Could you check a few things on this model? Use its own coordinates, in mm. A direction names the side the tool comes from. Give positions to 0.01 mm unless a question says otherwise; leave off trailing zeros. Order: outer loops, then holes, each group sorted by start corner. A loop starts at its lowest first (then second) coordinate and runs counter-clockwise, first axis right, second up. Notation, with made-up numbers: M 72,15.5 L 125,15.5 A20 ccw 125,21.5 Z; hole C -1.75,71 d11. An arc over 180 degrees is marked long. Answer in a Markdown table with one row per item. Add a question column.
```python
from build123d import *

# Parameters (mm, degrees)
SKETCH3_W           = 7.302665
SKETCH3_H           = 36.305572
FACE_CUT_DEPTH      = 10
LINK_ARMS_REACH     = 26.639
ROUNDED_LINKS_REACH = 32.365
SKETCH6_R           = 4
TRIM_1_REACH        = 35.167
SKETCH7_R           = 1.5
SKETCH8_W           = 8
SKETCH8_H           = 8.25
TRIM_2_DEPTH        = 15


with BuildPart() as part:
    # Sketch1 → Base Cylinder (revolve)
    with BuildSketch(Plane.XY, mode=Mode.PRIVATE) as base_cylinder_sk:
        with BuildLine():
            Line((-16, 2.5), (-16, 7.5))
            Line((-16, 7.5), (-12.5, 7.5))
            ThreePointArc((-12.5, 7.5), (-11.792893, 7.792893), (-11.5, 8.5))
            Line((-11.5, 8.5), (-11.5, 9.75))
            Line((-11.5, 9.75), (0, 9.75))
            Line((0, 9.75), (0, 8.25))
            Line((0, 8.25), (-3.5, 8.25))
            Line((-3.5, 8.25), (-3.5, 2.5))
            Line((-3.5, 2.5), (-16, 2.5))
        make_face()
    revolve(base_cylinder_sk.sketch.rotate(Axis((-29.02439, 0, 0), (1, 0, 0)), 90), axis=Axis((-29.02439, 0, 0), (1, 0, 0)))

    # Sketch2 → Suspension attachments (revolve)
    with BuildSketch(Plane(origin=(-3.375, 0, 0), x_dir=(0, 0, -1), z_dir=(1, 0, 0))):
        with BuildLine():
            Line((-3.375, 16), (-1.5, 16))
            Line((-1.5, 16), (-1.5, 9.633924))
            ThreePointArc((-1.5, 9.633924), (-3.80208, 8.978123), (-5.875, 7.781187))
            Line((-5.875, 7.781187), (-3.375, 12.111314))
            Line((-3.375, 12.111314), (-3.375, 16))
        make_face()
    suspension_attachments = revolve(axis=Axis((-3.375, 16.888615, 0), (0, -1, 0)))

    # Mirror1: Suspension attachments across plane
    add(suspension_attachments.mirror(Plane.ZX))

    # Sketch3 → Face Cut (cut, symmetric)
    with BuildSketch(Plane.XY):
        with Locations((3.651332, -0.216492)):
            Rectangle(SKETCH3_W, SKETCH3_H)
    extrude(amount=FACE_CUT_DEPTH, both=True, mode=Mode.SUBTRACT)

    # Link Arms: up to this face of the body (flat: up to its plane)
    link_arms_end = Plane(part.part.faces().sort_by_distance((-11.5, 0, -8.775772))[0])
    # Sketch5 → Link Arms (add, up to the picked face)
    with BuildSketch(Plane(origin=(0, 0, 0), x_dir=(0, 0, -1), z_dir=(1, 0, 0)), mode=Mode.PRIVATE) as link_arms_sk1:
        with BuildLine():
            Line((9.75, 0), (20.25, 0))
            Line((20.25, 0), (20.25, -2.5))
            Line((20.25, -2.5), (9.424038, -2.5))
            ThreePointArc((9.424038, -2.5), (9.668166, -1.26058), (9.75, 0))
        make_face()
    link_arms_tool1 = split(extrude(link_arms_sk1.sketch, amount=-LINK_ARMS_REACH, mode=Mode.PRIVATE), bisect_by=link_arms_end, keep=Keep.BOTH, mode=Mode.PRIVATE)
    # Sketch5 → Link Arms (add, up to the picked face)
    with BuildSketch(Plane(origin=(0, 0, 0), x_dir=(0, 0, -1), z_dir=(1, 0, 0)), mode=Mode.PRIVATE) as link_arms_sk2:
        with BuildLine():
            Line((5.887009, -7.772106), (11.044873, -10.75))
            Line((11.044873, -10.75), (20.25, -10.75))
            Line((20.25, -10.75), (20.25, -13.25))
            Line((20.25, -13.25), (10.375, -13.25))
            Line((10.375, -13.25), (3.309929, -9.17098))
            ThreePointArc((3.309929, -9.17098), (4.651358, -8.568977), (5.887009, -7.772106))
        make_face()
    link_arms_tool2 = split(extrude(link_arms_sk2.sketch, amount=-LINK_ARMS_REACH, mode=Mode.PRIVATE), bisect_by=link_arms_end, keep=Keep.BOTH, mode=Mode.PRIVATE)
    add(link_arms_tool1.solids().sort_by(Axis((0, -1.25638, -14.945599), (-1, 0, 0)))[0])
    add(link_arms_tool2.solids().sort_by(Axis((0, -11.294384, -12.172928), (-1, 0, 0)))[0])

    # Rounded Links: up to this face of the body (flat: up to its plane)
    rounded_links_end = Plane(part.part.faces().sort_by_distance((-5.75, -13.25, -15.3125))[0])
    # Sketch6 → Rounded Links (add, up to the picked face)
    with BuildSketch(Plane(origin=(0, 0, 0), x_dir=(1, 0, 0), z_dir=(0, 1, 0)), mode=Mode.PRIVATE) as rounded_links_sk1:
        with Locations(Location((-5.75, 20.25, 0), (0, 0, 180))):
            Circle(SKETCH6_R)
    rounded_links_tool1 = split(extrude(rounded_links_sk1.sketch, amount=-ROUNDED_LINKS_REACH, mode=Mode.PRIVATE), bisect_by=rounded_links_end, keep=Keep.BOTH, mode=Mode.PRIVATE)
    add(rounded_links_tool1.solids().sort_by(Axis((-5.75, 0, -20.25), (0, -1, 0)))[0])

    # Trim 1: up to this face of the body (flat: up to its plane)
    trim_1_end = Plane(part.part.faces().sort_by_distance((-5.75, -13.25, -16.514845))[0])
    # Sketch7 → Trim 1 (cut, up to the picked face)
    with BuildSketch(Plane(origin=(0, 0, 0), x_dir=(1, 0, 0), z_dir=(0, 1, 0)), mode=Mode.PRIVATE) as trim_1_sk1:
        with Locations(Location((-5.75, 20.25, 0), (0, 0, 270))):
            Circle(SKETCH7_R)
    trim_1_tool1 = split(extrude(trim_1_sk1.sketch, amount=-TRIM_1_REACH, mode=Mode.PRIVATE), bisect_by=trim_1_end, keep=Keep.BOTH, mode=Mode.PRIVATE)
    # Sketch7 → Trim 1 (cut, up to the picked face)
    with BuildSketch(Plane(origin=(0, 0, 0), x_dir=(1, 0, 0), z_dir=(0, 1, 0)), mode=Mode.PRIVATE) as trim_1_sk2:
        Polygon((-9.75, 20.25), (-11.5, 9.75), (-11.5, 20.25), align=None)
    trim_1_tool2 = split(extrude(trim_1_sk2.sketch, amount=-TRIM_1_REACH, mode=Mode.PRIVATE), bisect_by=trim_1_end, keep=Keep.BOTH, mode=Mode.PRIVATE)
    # Sketch7 → Trim 1 (cut, up to the picked face)
    with BuildSketch(Plane(origin=(0, 0, 0), x_dir=(1, 0, 0), z_dir=(0, 1, 0)), mode=Mode.PRIVATE) as trim_1_sk3:
        Polygon((-1.75, 20.25), (0, 9.75), (0, 20.25), align=None)
    trim_1_tool3 = split(extrude(trim_1_sk3.sketch, amount=-TRIM_1_REACH, mode=Mode.PRIVATE), bisect_by=trim_1_end, keep=Keep.BOTH, mode=Mode.PRIVATE)
    add(trim_1_tool1.solids().sort_by(Axis((-5.75, 0, -20.25), (0, -1, 0)))[0], mode=Mode.SUBTRACT)
    add(trim_1_tool2.solids().sort_by(Axis((-10.916667, 0, -16.75), (0, -1, 0)))[0], mode=Mode.SUBTRACT)
    add(trim_1_tool3.solids().sort_by(Axis((-0.583333, 0, -16.75), (0, -1, 0)))[0], mode=Mode.SUBTRACT)

    # Sketch8 → Trim 2 (cut, symmetric)
    with BuildSketch(Plane(origin=(1.581081, 0, -0.263514), x_dir=(-0.1643989873053571, 0, -0.9863939238321439), z_dir=(0.9863939238321439, 0, -0.1643989873053571))):
        with Locations((20.919771, -6.625)):
            Rectangle(SKETCH8_W, SKETCH8_H)
    extrude(amount=TRIM_2_DEPTH, both=True, mode=Mode.SUBTRACT)


solid = part.part
```
1. If I drill on line 1 along Y through (x, z) = (-3.75, 2); line 2 along Y through (x, z) = (-8, -21); line 3 along X through (y, z) = (-1.55, -20.25), over which ranges is the centre line in solid material (lowest first)? Write a range as [from, to].
2. Thinking about a two-plate mould opening in X: for faces 5 (the cylindrical face through (-3.36, 9.75, -0.03)), 6 (the flat face through (-16, -2, 2)), 7 (the cylindrical face through (-1.77, -2.48, 7.87)), which applies, pulls with the +X half, pulls with the -X half, needs draft (parallel to the pull), parting line crosses it, or undercut?
3. Will these pins go through, and if not, where does the flat tip stop? P1, Ø10, axis at y = -6.5, z = -14, coming from the +X side; P2, Ø19, axis at y = 0, z = 0, coming from the +X side; P3, Ø4, axis at x = -7, z = -15.5, coming from the -Y side; P4, Ø3, axis at x = -2.5, y = 4, coming from the +Z side.
4. For faces 1 (the flat face through (-11.5, -5.8, -6.5)), 2 (the cylindrical face through (-9.8, -0.1, -2.5)), 3 (the cylindrical face through (-3.4, -12.8, -1.5)), 4 (the flat face through (-3.5, 2, -2)), which set-ups out of +Z, -Z, +X, -X, +Y, -Y let a thin tool reach every point of the face, with its end or its side?
5. Suppose I cut it at A-A on z = -15. List the corners of the cut face in (x, y) for me (3 decimals).
6. Suppose I cut it at B-B on x = -13. List the corners of the cut face in (y, z) for me.
7. Suppose I cut it at D-D on x = -5.75. Count the separate pieces of the cut face and the enclosed holes in it, plus the area to 3 significant figures.
8. Suppose I cut it at C-C on y = 11. List the corners of the cut face in (x, z) for me (3 decimals), plus the area to 3 significant figures.
Findings below:
| question | item | result |
|---|---|---|
| 1 | line 1 | [-16, -1.5], [1.5, 16] |
| 1 | line 2 | [-13.25, -10.75], [-2.5, 0] |
| 1 | line 3 | [-9.75, -7.25], [-4.25, -1.75] |
| 2 | face 5 | undercut |
| 2 | face 6 | pulls with the -X half |
| 2 | face 7 | needs draft |
| 3 | P1 | x = -0.21 |
| 3 | P2 | x = 0 |
| 3 | P3 | y = -13.25 |
| 3 | P4 | z = 9.42 |
| 4 | face 1 | -X |
| 4 | face 2 | +X, -X |
| 4 | face 3 | -Y |
| 4 | face 4 | +X |
| 5 | outline | M -10.625,-13.25 L -0.875,-13.25 L -0.875,-10.75 L -10.625,-10.75 Z; M -10.625,-2.5 L -0.875,-2.5 L -0.875,0 L -10.625,0 Z |
| 6 | outline | C 0,0 d15; hole C 0,0 d5 |
| 7 | separate pieces | 3 |
| 7 | enclosed holes | 1 |
| 7 | area | 426 mm2 |
| 8 | outline | M 0,-2.178 L 0,2.178 A4.017 ccw long Z; hole C -3.375,0 d3 |
| 8 | area | 41.7 mm2 |
